```python
from build123d import *

# Parameters (mm, degrees)
F0_W     = 570
F0_H     = 170
F1_DEPTH = 30
F2_W     = 500
F2_H     = 150
F3_DEPTH = 10
F4_W     = 480
F4_H     = 130
F5_DEPTH = 20


with BuildPart() as f1:
    # F0 (on Top) → F1 (new body)
    with BuildSketch(Plane.XY):
        with Locations((11.190109, -17.617314)):
            Rectangle(F0_W, F0_H)
    extrude(amount=-F1_DEPTH)

    # F2 (on face) → F3 (cut)
    with BuildSketch(Plane.XY):
        with Locations((-13.809891, -17.617314)):
            Rectangle(F2_W, F2_H)
    extrude(amount=-F3_DEPTH, mode=Mode.SUBTRACT)

    # F4 (on face) → F5 (cut, through all)
    with BuildSketch(Plane.XY.offset(-10)):
        with Locations((-13.809891, -17.617314)):
            Rectangle(F4_W, F4_H)
    extrude(amount=-F5_DEPTH, mode=Mode.SUBTRACT)


solid = f1.part
```
Source: CAD feature listing. Evaluate the final solid. Frame: model axes, mm. A direction names the side the tool comes from. Give positions to 0.01 mm unless a question says otherwise; leave off trailing zeros. Order: outer loops, then holes, each group sorted by start corner. A loop starts at its lowest first (then second) coordinate and runs counter-clockwise, first axis right, second up. Notation, with made-up numbers: (15.5, 0) -> (71.5, 0) arc R17 ccw to (71.5, 28) -> close; hole circle Ø5 at (58, 65.25). An arc over 180 degrees is marked (long way). Use a Markdown table: item, result.
Q1. Section A-A (z = -16.25). Return the cut outline in (x, y), and give its area (3 significant figures).
A:
| item | result |
|---|---|
| outline | (-273.81, -102.62) -> (296.19, -102.62) -> (296.19, 67.38) -> (-273.81, 67.38) -> close; hole (-253.81, -82.62) -> (226.19, -82.62) -> (226.19, 47.38) -> (-253.81, 47.38) -> close |
| area | 34,500 mm^2 |
Q2. Access query for faces 1 (the face through (73, 58, 0)), 2 (the face through (-17, 57.383, -5)), 3 (the face through (-17, 47.383, -20)). Directions: +Z, -Z, +X, -X, +Y, -Y. A direction counts if a zero-diameter tool reaches every point of the face in a straight line with its end or side. Return the directions, or none.
A:
| item | result |
|---|---|
| face 1 | +Z, +X, -X, +Y, -Y |
| face 2 | +Z |
| face 3 | +Z, -Z |
Q3. Section C-C (y = -15.5). Return the cut outline in (x, z), and give its area (3 significant figures).
A:
| item | result |
|---|---|
| outline | (-273.81, -30) -> (-253.81, -30) -> (-253.81, -10) -> (-263.81, -10) -> (-263.81, 0) -> (-273.81, 0) -> close; (226.19, -30) -> (296.19, -30) -> (296.19, 0) -> (236.19, 0) -> (236.19, -10) -> (226.19, -10) -> close |
| area | 2,500 mm^2 |
Q4. Material intervals for line 1 (X direction, y = -71.5, z = -25.25); line 2 (Y direction, x = -210.5, z = -4); line 3 (Y direction, x = 212.5, z = -26.5), sorted ascending. Write a range as [from, to].
A:
| item | result |
|---|---|
| line 1 | [-273.81, -253.81], [226.19, 296.19] |
| line 2 | [-102.62, -92.62], [57.38, 67.38] |
| line 3 | [-102.62, -82.62], [47.38, 67.38] |
Q5. Section B-B (x = -181). Return the cut outline in (y, z), and give its area (3 significant figures).
A:
| item | result |
|---|---|
| outline | (-102.62, -30) -> (-82.62, -30) -> (-82.62, -10) -> (-92.62, -10) -> (-92.62, 0) -> (-102.62, 0) -> close; (47.38, -30) -> (67.38, -30) -> (67.38, 0) -> (57.38, 0) -> (57.38, -10) -> (47.38, -10) -> close |
| area | 1,000 mm^2 |
